```python
from build123d import *

# Parameters (mm, degrees)
F0_W     = 754.38
F0_H     = 533.4
F0_R     = 63.5
F2_DEPTH = 50.8
F3_DEPTH = 50.8
F4_DEPTH = 63.5


with BuildPart() as f2:
    # F0 (on Top) → F2 (new body)
    with BuildSketch(Plane.XY):
        Rectangle(F0_W, F0_H)
        Circle(F0_R, mode=Mode.SUBTRACT)
    extrude(amount=F2_DEPTH)

    # F1 (on Top) → F3 (join, through all)
    with BuildSketch(Plane.XY):
        Polygon((-389.89, -279.4), (-313.69, -279.4), (-313.69, -266.7), (-377.19, -266.7), (-377.19, -203.2), (-389.89, -203.2), align=None)
        Polygon((-313.69, 266.7), (-313.69, 279.4), (-389.89, 279.4), (-389.89, 203.2), (-377.19, 203.2), (-377.19, 266.7), align=None)
    extrude(amount=F3_DEPTH)

    # F1 (on Top) → F4 (join)
    with BuildSketch(Plane.XY):
        Polygon((389.89, -203.2), (377.19, -203.2), (377.19, -266.7), (313.69, -266.7), (313.69, -279.4), (389.89, -279.4), align=None)
        Polygon((377.19, 266.7), (377.19, 203.2), (389.89, 203.2), (389.89, 279.4), (313.69, 279.4), (313.69, 266.7), align=None)
    extrude(amount=F4_DEPTH)


solid = f2.part
```
For this review, take the finished solid that the model builds, in its own axes (mm). A direction names the side the tool comes from. Coordinates: 2 decimals unless noted, no trailing zeros. Order: outer loops, then holes, each group sorted by start corner. A loop starts at its lowest first (then second) coordinate and runs counter-clockwise, first axis right, second up. Notation, with made-up numbers: (56.25, 79.5) -> (99.25, 79.5) arc R4 cw to (99.25, 85.5) -> close; hole circle Ø6 at (59, -32.5). An arc over 180 degrees is marked (long way). Use CSV: the item, a comma, the result in double quotes. Start each with the question number.
Item 1: Insertion check: pin 1 (6 mm diameter, centred on x = -204.5, y = -143, fed in from +Z); pin 2 (3 mm diameter, centred on x = 216.5, y = -84.5, fed in from -Z); pin 3 (1.5 mm diameter, centred on y = 101.5, z = 51.5, fed in from +X); pin 4 (8 mm diameter, centred on x = 275, z = 39.5, fed in from +Y). Each pin has a flat end and moves straight along its axis. Give the tip position at first contact, or say it passes through.
Item 2: We need section D-D, the plane y = 180.5. Give the boundary of the cut face in (x, z), then the cut area to 3 significant figures.
Item 3: Wall thickness on probe 1 along Y at (x, z) = (0, 12); probe 2 along Z at (x, y) = (-106, -138); probe 3 along Y at (x, z) = (-106, 45.5): over which ranges is each line inside the solid? List them lowest first.
Item 4: For faces 5 (the face through (363, 273, 63.5)), 6 (the face through (-377.19, -3, 25)), 7 (the face through (377.19, -3, 25)), list the 3-axis set-ups (+Z, -Z, +X, -X, +Y, -Y) from which the entire face can be reached by the end or side of a thin tool; tool diameter is ignored.
Item 5: We need section C-C, the plane y = 0. Give the boundary of the cut face in (x, z), then the cut area to 3 significant figures.
Item 6: Draft analysis for pull direction X (two halves, no side actions). For faces 1 (the face through (-4, -266.7, 25)), 2 (the face through (-389.89, -241, 25)), 3 (the face through (-5, 66, 0)), 4 (the face through (-4, 266.7, 25)), state which applies: pulls with the +X half, pulls with the -X half, needs draft (parallel to the pull), parting line crosses it, or undercut.
Item 7: We need section A-A, the plane x = 0. Give the boundary of the cut face in (y, z), then the cut area to 3 significant figures.
Item 8: We need section B-B, the plane z = 14.5. Give the boundary of the cut face in (x, y).
Derived:
1,pin 1,"stops at z = 50.8"
1,pin 2,"stops at z = 0"
1,pin 3,"stops at x = 377.19"
1,pin 4,"stops at y = 266.7"
2,outline,"(-377.19, 0) -> (377.19, 0) -> (377.19, 50.8) -> (-377.19, 50.8) -> close"
2,area,"38,300 mm^2"
3,probe 1,"y = -266.7 to -63.5, 63.5 to 266.7"
3,probe 2,"z = 0 to 50.8"
3,probe 3,"y = -266.7 to 266.7"
4,face 5,"+Z, +X, -X, +Y, -Y"
4,face 6,"+Z, -Z, -X"
4,face 7,"+Z, -Z, +X"
5,outline,"(-377.19, 0) -> (-63.5, 0) -> (-63.5, 50.8) -> (-377.19, 50.8) -> close; (63.5, 0) -> (377.19, 0) -> (377.19, 50.8) -> (63.5, 50.8) -> close"
5,area,"31,900 mm^2"
6,face 1,"undercut"
6,face 2,"pulls with the -X half"
6,face 3,"needs draft"
6,face 4,"undercut"
7,outline,"(-266.7, 0) -> (-63.5, 0) -> (-63.5, 50.8) -> (-266.7, 50.8) -> close; (63.5, 0) -> (266.7, 0) -> (266.7, 50.8) -> (63.5, 50.8) -> close"
7,area,"20,600 mm^2"
8,outline,"(-389.89, -279.4) -> (-313.69, -279.4) -> (-313.69, -266.7) -> (313.69, -266.7) -> (313.69, -279.4) -> (389.89, -279.4) -> (389.89, -203.2) -> (377.19, -203.2) -> (377.19, 203.2) -> (389.89, 203.2) -> (389.89, 279.4) -> (313.69, 279.4) -> (313.69, 266.7) -> (-313.69, 266.7) -> (-313.69, 279.4) -> (-389.89, 279.4) -> (-389.89, 203.2) -> (-377.19, 203.2) -> (-377.19, -203.2) -> (-389.89, -203.2) -> close; hole circle Ø127 at (0, 0)"
